```python
from build123d import *

# Parameters (mm, degrees)
BOSS_EXTRUDE1_DEPTH = 11.8
BOSS_EXTRUDE2_DEPTH = 4
SKETCH4_R           = 2.3
BOSS_EXTRUDE3_DEPTH = 3.2
CUT_EXTRUDE1_DEPTH  = 3.2
CUT_EXTRUDE2_DEPTH  = 3.2


with BuildPart() as part:
    # Sketch2 → Boss-Extrude1 (new body)
    with BuildSketch(Plane.XY):
        Polygon((0, 0), (22.5, 0), (22.5, 15.9), (27.2, 15.9), (27.2, 18.4), (22.5, 18.4), (22.5, 22.7), (0, 22.7), (0, 18.4), (-4.7, 18.4), (-4.7, 15.9), (0, 15.9), align=None)
    extrude(amount=BOSS_EXTRUDE1_DEPTH)

    # Sketch3 → Boss-Extrude2 (add)
    with BuildSketch(Plane(origin=(0, 22.7, 0), x_dir=(1, 0, 0), z_dir=(0, 1, 0))):
        with BuildLine():
            ThreePointArc((11.270338983, -3.456752324), (0, -5.9), (11.270338983, -8.343247676))
            ThreePointArc((11.270338983, -8.343247676), (14.3, -5.9), (11.270338983, -3.456752324))
        make_face()
    extrude(amount=BOSS_EXTRUDE2_DEPTH)

    # Sketch4 → Boss-Extrude3 (add)
    with BuildSketch(Plane(origin=(0, 26.7, 0), x_dir=(1, 0, 0), z_dir=(0, 1, 0))):
        with Locations((5.9, -5.9)):
            Circle(SKETCH4_R)
    extrude(amount=BOSS_EXTRUDE3_DEPTH)

    # Sketch5 → Cut-Extrude1 (cut)
    with BuildSketch(Plane(origin=(0, 18.4, 0), x_dir=(1, 0, 0), z_dir=(0, 1, 0))):
        with BuildLine():
            Line((27.2, -5.9), (27.2, -5.25))
            Line((27.2, -5.25), (25.659934208, -5.25))
            ThreePointArc((25.659934208, -5.25), (23.9, -5.9), (25.659934208, -6.55))
            Line((25.659934208, -6.55), (27.2, -6.55))
            Line((27.2, -6.55), (27.2, -5.9))
        make_face()
    extrude(amount=-CUT_EXTRUDE1_DEPTH, mode=Mode.SUBTRACT)

    # Sketch6 → Cut-Extrude2 (cut)
    with BuildSketch(Plane(origin=(0, 18.4, 0), x_dir=(1, 0, 0), z_dir=(0, 1, 0))):
        with BuildLine():
            Line((-4.7, -5.9), (-4.7, -5.25))
            Line((-4.7, -5.25), (-3.159934208, -5.25))
            ThreePointArc((-3.159934208, -5.25), (-1.4, -5.9), (-3.159934208, -6.55))
            Line((-3.159934208, -6.55), (-4.7, -6.55))
            Line((-4.7, -6.55), (-4.7, -5.9))
        make_face()
    extrude(amount=-CUT_EXTRUDE2_DEPTH, mode=Mode.SUBTRACT)


solid = part.part
```
Can you work these out from the model? Positions are in its coordinate system, mm. A direction names the side the tool comes from. Round coordinates to 2 decimals unless told otherwise and drop trailing zeros. Order: outer loops, then holes, each group sorted by start corner. A loop starts at its lowest first (then second) coordinate and runs counter-clockwise, first axis right, second up.
(1) If we section it at C-C (y = 17): Please give me the cut outline in (x, z), plus the area to 3 significant figures.
Results are:
outline: (-4.7, 0) - (27.2, 0) - (27.2, 5.25) - (25.66, 5.25) arc R1 cw (long way) to (25.66, 6.55) - (27.2, 6.55) - (27.2, 11.8) - (-4.7, 11.8) - (-4.7, 6.55) - (-3.16, 6.55) arc R1 cw (long way) to (-3.16, 5.25) - (-4.7, 5.25) - close
area: 367 mm2
(2) I'm going to push flat-ended pins straight in: pin 1 (2 mm diameter, centred on y = 20, z = 10, fed in from -X); pin 2 (3 mm diameter, centred on x = -2.4, z = 5.9, fed in from +Y); pin 3 (6 mm diameter, centred on x = 12, z = 8, fed in from +Y). Where does each tip first touch, or does it pass through?
Results are:
pin 1: stops at x = 0
pin 2: stops at y = 18.4
pin 3: stops at y = 26.7
(3) If we section it at D-D (z = 7.75): Please give me the cut outline in (x, y).
Results are:
outline: (-4.7, 15.9) - (0, 15.9) - (0, 0) - (22.5, 0) - (22.5, 15.9) - (27.2, 15.9) - (27.2, 18.4) - (22.5, 18.4) - (22.5, 22.7) - (13.48, 22.7) - (13.48, 26.7) - (7.27, 26.7) - (7.27, 29.9) - (4.53, 29.9) - (4.53, 26.7) - (0.3, 26.7) - (0.3, 22.7) - (0, 22.7) - (0, 18.4) - (-4.7, 18.4) - close
(4) If we section it at A-A (x = -2.4): Please give me the cut outline in (y, z), plus the area to 3 significant figures.
Results are:
outline: (15.9, 0) - (18.4, 0) - (18.4, 4.9) - (15.9, 4.9) - close; (15.9, 6.9) - (18.4, 6.9) - (18.4, 11.8) - (15.9, 11.8) - close
area: 24.5 mm2
(5) We'd pull the mould along Z, two halves only. Please class faces 5 (the face through (9, 26.7, 6)), 6 (the face through (-4, 17, 5.25)), 7 (the face through (14.3, 24.7, 6)): +Z half, -Z half, draft (parallel to the pull), parting line (faces both ways), or undercut.
Results are:
face 5: draft
face 6: undercut
face 7: parting line
(6) If we section it at B-B (x = 11.8): Please give me the cut outline in (y, z).
Results are:
outline: (0, 0) - (22.7, 0) - (22.7, 3.4) - (26.7, 3.4) - (26.7, 8.4) - (22.7, 8.4) - (22.7, 11.8) - (0, 11.8) - close
(7) If I drill on L1, parallel to Z at x = -2.4, y = 17.25; L2, parallel to Y at x = 8, z = 10; L3, parallel to Y at x = -1.5, z = 3.5, over which ranges is the centre line in solid material (lowest first)?
Results are:
L1: z = 0 to 4.9, 6.9 to 11.8
L2: y = 0 to 26.7
L3: y = 15.9 to 18.4
(8) On a 3-axis mill with a long thin cutter (end or side, diameter ignored), from which of +Z, -Z, +X, -X, +Y, -Y can I reach the whole of each face in a straight line? I mean faces 1 (the face through (22.5, 8, 6)), 2 (the face through (24.9, 18.4, 4.5)), 3 (the face through (26, 17, 6.55)), 4 (the face through (-1, 15.9, 6)). Say none if no direction works.
Results are:
face 1: +Z, -Z, +X, -Y
face 2: +Z, -Z, +X, +Y
face 3: +X, +Y, -Y
face 4: +Z, -Z, -X, -Y
